Could you check a few things on this model? Use its own coordinates, in mm. A direction names the side the tool comes from. Round coordinates to 2 decimals unless told otherwise and drop trailing zeros. Loops run counter-clockwise (first coordinate to the right, second up) from the corner with the lowest first, then second, coordinate; pieces in that order, holes last. Notation, with made-up numbers: (-9.75, 77) -> (18.25, 77) arc R23 ccw to (18.25, 107) -> close; hole circle Ø4 at (-14.75, 89.25). An arc over 180 degrees is marked (long way). One line per item, written item: value.
```python
from build123d import *

# Parameters (mm, degrees)
SKETCH_1_W      = 16.5
SKETCH_1_H      = 7
SKETCH_1_W_2    = 3.5
SKETCH_1_W_3    = 15
EXTRUDE_1_DEPTH = 100


with BuildPart() as part:
    # Эскиз1 → Бобышка-Вытянуть1 (new body)
    with BuildSketch(Plane.XY):
        with Locations((-11.75, 3.5)):
            Rectangle(SKETCH_1_W, SKETCH_1_H)
        with Locations((-1.75, 3.5)):
            Rectangle(SKETCH_1_W_2, SKETCH_1_H)
        Polygon((-3.5, 0), (-3.5, -16), (3.5, -16), (3.5, -9), (3.5, 16), (-3.5, 16), (-3.5, 7), (0, 7), (0, 0), align=None)
        with Locations((11, -12.5)):
            Rectangle(SKETCH_1_W_3, SKETCH_1_H)
    extrude(amount=EXTRUDE_1_DEPTH)


solid = part.part
```
Item 1: For faces 1 (the face through (-12, 7, 49)), 2 (the face through (-1, -3, 0)), 3 (the face through (-12, 0, 49)), 4 (the face through (3.5, 3, 49)), which set-ups out of +Z, -Z, +X, -X, +Y, -Y let a thin tool reach every point of the face, with its end or its side?
Output:
face 1: +Z, -Z, -X, +Y
face 2: -Z, +X, -X, +Y, -Y
face 3: +Z, -Z, -X, -Y
face 4: +Z, -Z, +X, +Y
Item 2: I need wall thicknesses on line 1 (Y direction, x = -17, z = 28.5); line 2 (Y direction, x = 13, z = 50); line 3 (X direction, y = 8.5, z = 28). Which ranges of each line are inside material? Lowest first, please. Write a range as from..to.
Output:
line 1: y = 0..7
line 2: y = -16..-9
line 3: x = -3.5..3.5
Item 3: If we section it at B-B on x = 8: List the corners of the cut face in (y, z) for me.
Output:
outline: (-16, 0) -> (-9, 0) -> (-9, 100) -> (-16, 100) -> close
Item 4: If we section it at A-A on z = 61.5: List the corners of the cut face in (x, y) for me.
Output:
outline: (-20, 0) -> (-3.5, 0) -> (-3.5, -16) -> (18.5, -16) -> (18.5, -9) -> (3.5, -9) -> (3.5, 16) -> (-3.5, 16) -> (-3.5, 7) -> (-20, 7) -> close
Item 5: If we section it at C-C on y = 6: List the corners of the cut face in (x, z) for me, plus the area to 3 significant figures.
Output:
outline: (-20, 0) -> (3.5, 0) -> (3.5, 100) -> (-20, 100) -> close
area: 2,350 mm²
Item 6: Will these pins go through, and if not, where does the flat tip stop? pin 1 Ø13 at (y, z) = (-11.5, 34) entering from -X; pin 2 Ø1.5 at (x, z) = (6, 24.5) entering from +Y; pin 3 Ø18 at (x, z) = (-14.5, 69.5) entering from -Y.
Output:
pin 1: stops at x = -3.5
pin 2: stops at y = -9
pin 3: stops at y = 0
